from build123d import *
from build123d.topology import SkipClean

# Parameters (mm, degrees)
SKETCH1_R           = 2
BOSS_EXTRUDE1_DEPTH = 3


with BuildPart() as part:
    # Sketch1 → Boss-Extrude1 (new body)
    with BuildSketch(Plane(origin=(0, 0, 0), x_dir=(1, 0, 0), z_dir=(0, 1, 0))):
        Polygon((-1.962990915, -3.4), (1.962990915, -3.4), (3.92598183, 0), (1.962990915, 3.4), (-1.962990915, 3.4), (-3.92598183, 0), align=None)
        with Locations(Location((0, 0, 0), (0, 0, 270))):
            Circle(SKETCH1_R, mode=Mode.SUBTRACT)
    extrude(amount=BOSS_EXTRUDE1_DEPTH)

    # Sketch2 → Revolve1 (revolve)
    with SkipClean():  # the faces are left unmerged after this step: merging them gives an invalid solid
        with BuildSketch(Plane(origin=(0, 0, 0), x_dir=(0, 0, -1), z_dir=(1, 0, 0)), mode=Mode.PRIVATE) as revolve1_sk:
            with BuildLine():
                Line((-2, 3), (-2, 5))
                Line((-2, 5), (-3, 5))
                ThreePointArc((-3, 5), (-3.299019514, 4.019803903), (-3.4, 3))
                Line((-3.4, 3), (-2, 3))
            make_face()
        revolve(revolve1_sk.sketch.rotate(Axis((0, 0, 0), (0, 1, 0)), 180), axis=Axis((0, 0, 0), (0, 1, 0)))
    add(part.part.scale(1), mode=Mode.REPLACE)  # the faces are merged on a copy


solid = part.part
Input: part model. Units: mm. Frame: model coordinates. A direction names the side the tool comes from. Round coordinates to 2 decimals unless told otherwise and drop trailing zeros. Order: outer loops, then holes, each group sorted by start corner. A loop starts at its lowest first (then second) coordinate and runs counter-clockwise, first axis right, second up.
1. Set-up query: faces 1 (the face through (-2, 3, -3)), 2 (the face through (2, 3, -3)), 3 (the face through (2, 3, 3)), 4 (the face through (-2, 3, 3)), 5 (the face through (-2.958, 1.479, 1.676)). Return all of +Z, -Z, +X, -X, +Y, -Y with unobstructed straight access to the full face (end or side cutting, diameter ignored); none if empty.
The answers:
face 1: -Z, -X, +Y
face 2: -Z, +X, +Y
face 3: +Z, +X, +Y
face 4: +Z, -X, +Y
face 5: +Z, -X, +Y, -Y
2. Pin query (flat end, axial travel): P1, Ø3, axis at y = 1.5, z = 2.5, coming from the +X side; P2, Ø1.1, axis at x = -3, z = -0.5, coming from the +Y side. Return the tip coordinate at first contact, or that it passes through.
The answers:
P1: stops at x = 3.35
P2: stops at y = 5
3. Material intervals for line 1 (Z direction, x = -1.75, y = 1.4); line 2 (Z direction, x = -0.75, y = 1.95); line 3 (X direction, y = 4.2, z = 0), sorted ascending.
The answers:
line 1: z = -3.4 to -0.97, 0.97 to 3.4
line 2: z = -3.4 to -1.85, 1.85 to 3.4
line 3: x = -3.26 to -2, 2 to 3.26
4. Cut plane A-A, the plane y = 0.95. Output: boundary loops of the cut face in (x, z).
The answers:
outline: (-3.93, 0) - (-1.96, -3.4) - (1.96, -3.4) - (3.93, 0) - (1.96, 3.4) - (-1.96, 3.4) - close; hole circle Ø4 at (0, 0)
